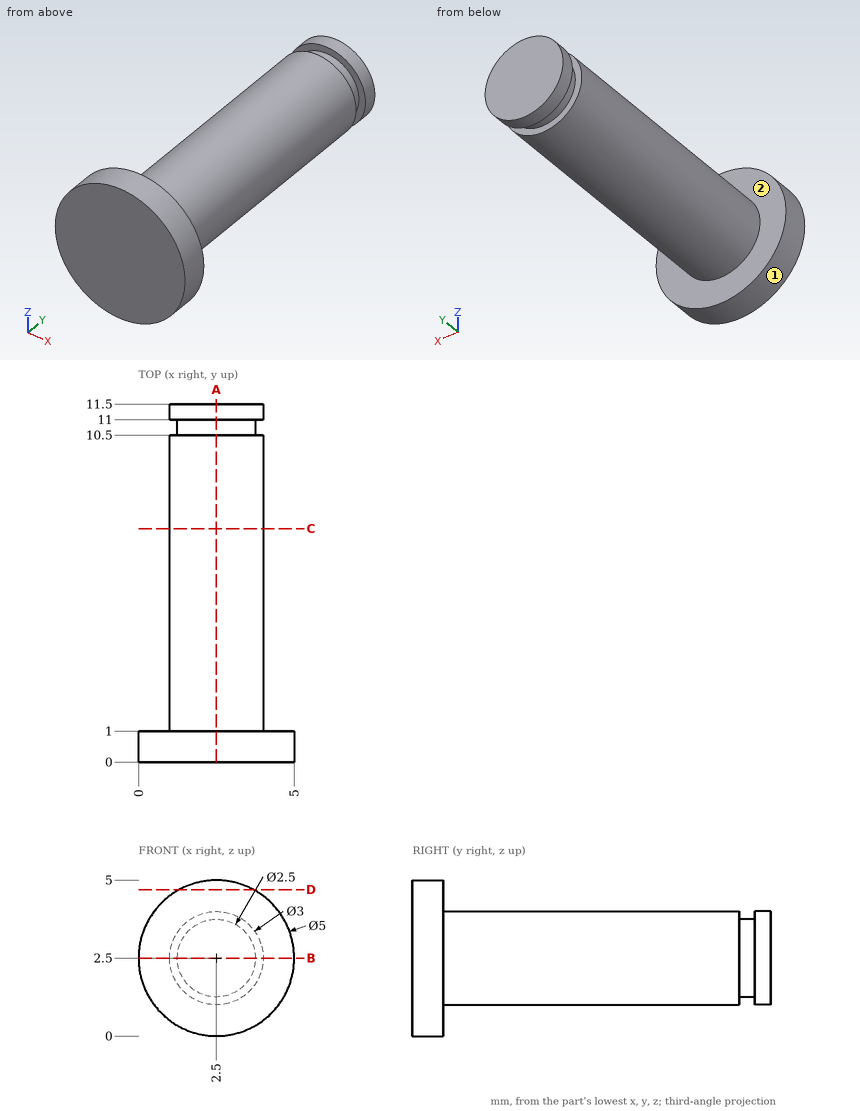
The figure shows three views and two pictorial views of one solid part (mm, origin at its lowest corner). Answer the questions. A direction names the side the tool comes from. Give positions to 0.01 mm unless a question says otherwise; leave off trailing zeros. Order: outer loops, then holes, each group sorted by start corner. A loop starts at its lowest first (then second) coordinate and runs counter-clockwise, first axis right, second up. Notation, with made-up numbers: (7, -37) - (53, -37) arc R23 cw to (53, -18) - close; hole circle Ø2 at (64.5, -13.75). An arc over 180 degrees is marked (long way). Answer as CSV lines item,"result".
Q1. Each of these flat-tipped pins is pushed along its axis until it touches: pin 1 Ø1.5 at (x, z) = (3, 3) entering from -Y; pin 2 Ø3 at (y, z) = (4.5, 2) entering from -X; pin 3 Ø2 at (y, z) = (5.5, 4.5) entering from +X; pin 4 Ø1 at (x, y) = (4, 5.5) entering from -Z. Where does it stop, or does it pass through?
Answer key:
pin 1,"stops at y = 0"
pin 2,"stops at x = 1"
pin 3,"stops at x = 3.62"
pin 4,"stops at z = 1.38"
Q2. Straight lines are drawn through the part: L1, parallel to Y at x = 3.7, z = 1.65; L2, parallel to Z at x = 2.45, y = 7.75; L3, parallel to Y at x = 2, z = 4. For each, find the intervals that lie inside material, in ascending order.
Answer key:
L1,"y = 0 to 10.5, 11 to 11.5"
L2,"z = 1 to 4"
L3,"y = 0 to 1"
Q3. Which of the six approach directions +Z, -Z, +X, -X, +Y, -Y give full straight-line access (tool end or side, diameter ignored) to the marked faces 1 and 2?
Answer key:
face 1,"+Y, -Y"
face 2,"+Y"
Q4. A cutting plane is placed at A-A, the plane x = 2.5. Determine the outline of the cut face in (y, z).
Answer key:
outline,"(0, 0) - (1, 0) - (1, 1) - (10.5, 1) - (10.5, 1.25) - (11, 1.25) - (11, 1) - (11.5, 1) - (11.5, 4) - (11, 4) - (11, 3.75) - (10.5, 3.75) - (10.5, 4) - (1, 4) - (1, 5) - (0, 5) - close"
Q5. A cutting plane is placed at D-D, the plane z = 4.7. Determine the outline of the cut face in (x, y).
Answer key:
outline,"(1.31, 0) - (3.69, 0) - (3.69, 1) - (1.31, 1) - close"
Q6. A cutting plane is placed at C-C, the plane y = 7.5. Determine the outline of the cut face in (x, z).
Answer key:
outline,"circle Ø3 at (2.5, 2.5)"
Q7. A cutting plane is placed at B-B, the plane z = 2.5. Determine the outline of the cut face in (x, y), and give its area (4 significant figures).
Answer key:
outline,"(0, 0) - (5, 0) - (5, 1) - (4, 1) - (4, 10.5) - (3.75, 10.5) - (3.75, 11) - (4, 11) - (4, 11.5) - (1, 11.5) - (1, 11) - (1.25, 11) - (1.25, 10.5) - (1, 10.5) - (1, 1) - (0, 1) - close"
area,"36.25 mm^2"
